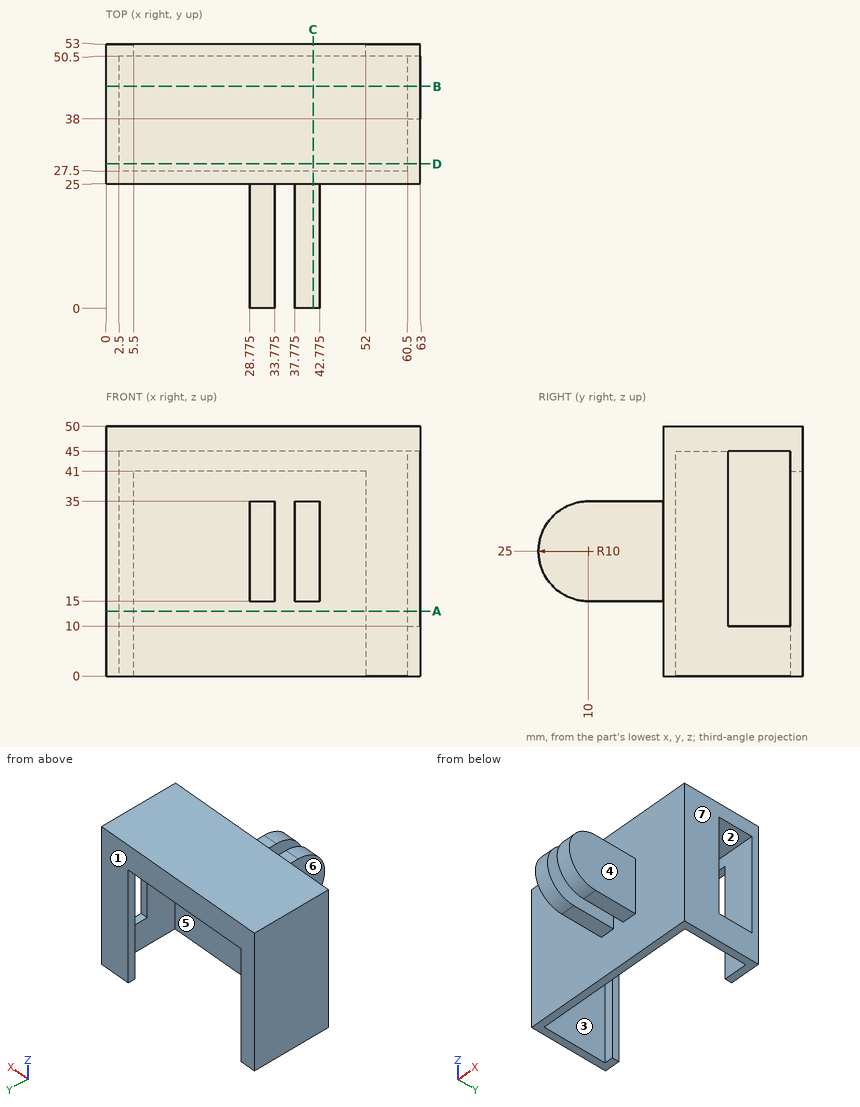
Print and shaded views of the part. All mm, measured from the part's lowest x, y and z. A direction names the side the tool comes from. Coordinates: 2 decimals unless noted, no trailing zeros. Write each loop counter-clockwise with the first axis right and the second up, starting at its lowest first coordinate (ties: lowest second). Pieces come first, ordered by that corner, then holes. Notation, with made-up numbers: M 29.25,0 L 51.25,0 A19 ccw 51.25,31 Z; hole C 60,-10.5 d9. An arc over 180 degrees is marked long. Return JSON: item names as keys, results as strings.
1. 3-axis set-ups, long thin cutter, end or side, ignore diameter. For the marked faces 5, 6 and 7: which of +Z, -Z, +X, -X, +Y, -Y reach the whole face in a straight line?
Determined:
{"face 5": "-Z", "face 6": "+Z, -Z, -X, -Y", "face 7": "+Z, -Z, +X, +Y, -Y"}
2. Saw through at D-D, the plane y = 29. Write the cut outline in (x, z).
Determined:
{"outline": "M 0,0 L 2.5,0 L 2.5,45 L 60.5,45 L 60.5,0 L 63,0 L 63,50 L 0,50 Z"}
3. Saw through at C-C, the plane x = 41.5. Write the cut outline in (y, z).
Determined:
{"outline": "M 10,15 L 25,15 L 25,0 L 27.5,0 L 27.5,45 L 50.5,45 L 50.5,41 L 53,41 L 53,50 L 25,50 L 25,35 L 10,35 A10 ccw Z"}
4. Pull direction Y, two halves, no side cores. Call the marked faces 1, 2, 3 and 4: pulls with the +Y half, pulls with the -Y half, needs draft (parallel to the pull), parting line crosses it, or undercut.
Determined:
{"face 1": "pulls with the +Y half", "face 2": "undercut", "face 3": "undercut", "face 4": "needs draft"}
5. Saw through at A-A, the plane z = 13. Write the cut outline in (x, y).
Determined:
{"outline": "M 0,25 L 63,25 L 63,38 L 60.5,38 L 60.5,27.5 L 2.5,27.5 L 2.5,50.5 L 5.5,50.5 L 5.5,53 L 0,53 Z; M 52,50.5 L 63,50.5 L 63,53 L 52,53 Z"}
6. Flat gauge pins, fed straight in: pin 1 Ø6 at (y, z) = (9, 22.5) entering from +X (3 decimals); pin 2 Ø11.5 at (x, y) = (36, 41) entering from -Z; pin 3 Ø5.5 at (x, y) = (30.5, 17.5) entering from +Z. Where does each tip first touch, or does it go through?
Determined:
{"pin 1": "x = 42.775", "pin 2": "z = 45", "pin 3": "z = 35"}
7. Probe L1, parallel to Y at x = 53, z = 21; L2, parallel to X at y = 3.5, z = 29 (1 decimal); L3, parallel to Y at x = 7.5, z = 11. List the from-to ranges inside material, lowest first.
Determined:
{"L1": "25 to 27.5, 50.5 to 53", "L2": "28.8 to 33.8, 37.8 to 42.8", "L3": "25 to 27.5"}
8. Saw through at B-B, the plane y = 44.5. Write the cut outline in (x, z).
Determined:
{"outline": "M 0,0 L 2.5,0 L 2.5,45 L 63,45 L 63,50 L 0,50 Z; M 60.5,0 L 63,0 L 63,10 L 60.5,10 Z"}
